Design review of the part shown in the three views and the two pictorial views. Dimensions are in mm from the part's minimum x, y and z. Coordinates: 2 decimals unless noted, no trailing zeros. Write each loop counter-clockwise with the first axis right and the second up, starting at its lowest first coordinate (ties: lowest second). Pieces come first, ordered by that corner, then holes. Notation, with made-up numbers: (-25, -4) - (-11, -4) arc R18 cw to (-11, 1) - close; hole circle Ø4 at (36, 3). An arc over 180 degrees is marked (long way). Write each question's results on one line, items separated by ' | '.
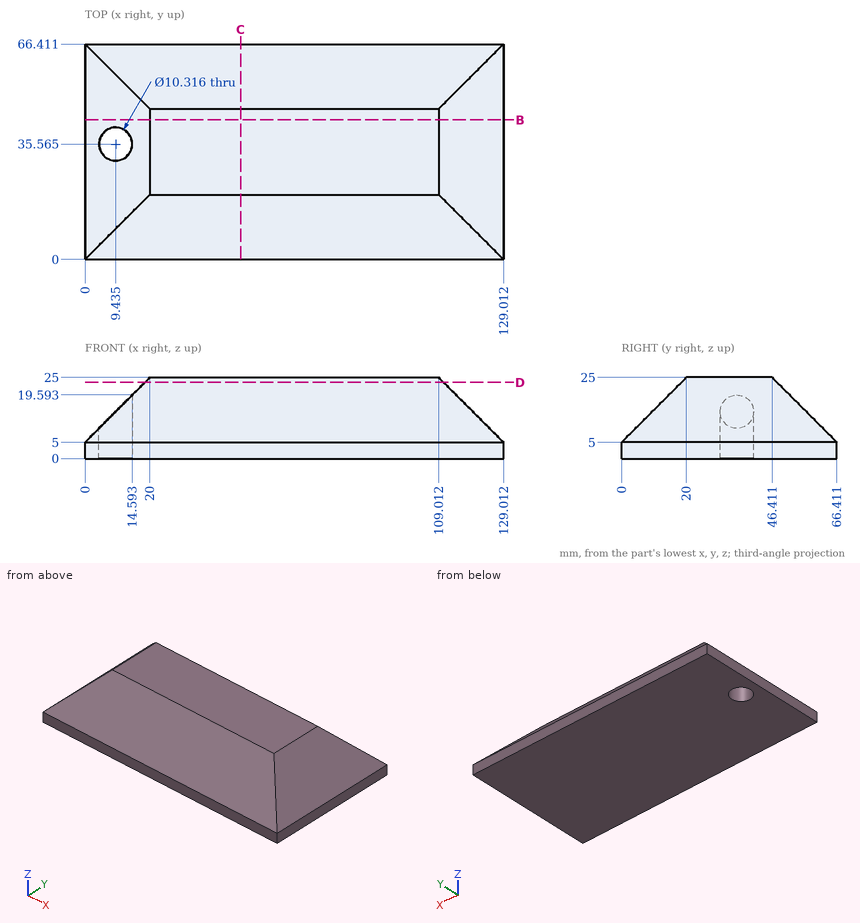
Q1. Take a section at B-B on y = 43. State the section outline as (x, z) points, plus the area to 3 significant figures.
Results found:
outline: (0, 0) - (129.01, 0) - (129.01, 5) - (109.01, 25) - (20, 25) - (0, 5) - close | area: 2,830 mm2
Q2. Wall thickness on line 1 along X through (y, z) = (33, 3.5); line 2 along X through (y, z) = (48.5, 16.5) (1 decimal); line 3 along Y through (x, z) = (45, 22.75): over which ranges is each line inside the solid? List them lowest first. Write a range as from..to.
Results found:
line 1: 0..4.96, 13.91..129.01 | line 2: 11.5..117.5 | line 3: 17.75..48.66
Q3. Take a section at D-D on z = 23.5. State the section outline as (x, y) points, plus the area to 3 significant figures.
Results found:
outline: (18.5, 18.5) - (110.51, 18.5) - (110.51, 47.91) - (18.5, 47.91) - close | area: 2,710 mm2
Q4. For pin 1 (12 mm diameter, centred on x = 61, z = 9.5, fed in from -Y); pin 2 (2 mm diameter, centred on y = 12.5, z = 8.5, fed in from -X); pin 3 (1 mm diameter, centred on y = 9.5, z = 7.5, fed in from -X); pin 4 (1 mm diameter, centred on x = 27, y = 9, fed in from +Z), all flat-tipped, find the tip position at first contact; note any pin that passes through.
Results found:
pin 1: y = 0 | pin 2: x = 2.5 | pin 3: x = 2 | pin 4: z = 14.5
Q5. Take a section at C-C on x = 48. State the section outline as (y, z) points, plus the area to 3 significant figures.
Results found:
outline: (0, 0) - (66.41, 0) - (66.41, 5) - (46.41, 25) - (20, 25) - (0, 5) - close | area: 1,260 mm2
